Source: CAD feature listing. Evaluate the final solid. Frame: model axes, mm. A direction names the side the tool comes from. Give positions to 0.01 mm unless a question says otherwise; leave off trailing zeros. Order: outer loops, then holes, each group sorted by start corner. A loop starts at its lowest first (then second) coordinate and runs counter-clockwise, first axis right, second up. Notation, with made-up numbers: (-15, -1.5) - (14, -1.5) arc R14 cw to (14, 9.5) - close; hole circle Ø4 at (-27.75, 89). An arc over 180 degrees is marked (long way). Use CSV: the item, a comma, the result in double quotes.
```python
from build123d import *

# Parameters (mm, degrees)
CHAMFER_SIZE    = 0.5
CHAMFER001_SIZE = 1
CHAMFER002_SIZE = 0.5
SKETCH001_W     = 2
SKETCH001_H     = 21.821188
POCKET_DEPTH    = 18.001


with BuildPart() as part:
    # Sketch → Revolution (revolve)
    with BuildSketch(Plane.XZ):
        Polygon((12.9, 0), (17.9, 0), (17.9, 12), (14.9, 12), (14.9, 18), (12.9, 18), align=None)
    revolve(axis=Axis((0, 0, 0), (0, 0, 1)))

    # Chamfer
    chamfer_edges = [part.edges().sort_by_distance(p)[0] for p in [
        (-14.9, 0, 12),
    ]]
    chamfer(chamfer_edges, length=CHAMFER_SIZE)

    # Chamfer001
    chamfer001_edges = [part.edges().sort_by_distance(p)[0] for p in [
        (-14.9, 0, 18),
    ]]
    chamfer(chamfer001_edges, length=CHAMFER001_SIZE)

    # Chamfer002
    chamfer002_edges = [part.edges().sort_by_distance(p)[0] for p in [
        (-12.9, 0, 0),
    ]]
    chamfer(chamfer002_edges, length=CHAMFER002_SIZE)

    # Sketch001 (on Face4 of Chamfer002) → Pocket (cut, through all)
    with BuildSketch(Plane(origin=(0, 0, 0), x_dir=(1, 0, 0), z_dir=(0, 0, -1))):
        with Locations((-0.050035, -17.700875)):
            Rectangle(SKETCH001_W, SKETCH001_H)
    extrude(amount=-POCKET_DEPTH, mode=Mode.SUBTRACT)


solid = part.part
```
Item 1: Section A-A on x = 0. Return the cut outline in (y, z), then the cut area to 3 significant figures.
Filled in:
outline,"(-17.9, 0) - (-13.4, 0) - (-12.9, 0.5) - (-12.9, 18) - (-13.9, 18) - (-14.9, 17) - (-14.9, 12.5) - (-15.4, 12) - (-17.9, 12) - close"
area,"71.5 mm2"
Item 2: Section B-B on z = 4. Return the cut outline in (x, y).
Filled in:
outline,"(-1.05, 12.86) - (-1.05, 17.87) arc R17.9 ccw (long way) to (0.95, 17.87) - (0.95, 12.86) arc R12.9 cw (long way) to start"
Item 3: First-contact query: pin 1 (1 mm diameter, centred on y = 13.5, z = 10, fed in from -X); pin 2 (4 mm diameter, centred on x = -9.5, y = -6, fed in from -Z); pin 3 (6 mm diameter, centred on y = 9.5, z = 14, fed in from -X). Flat tips, straight axial feed; report the tip coordinate or a pass-through.
Filled in:
pin 1,"stops at x = -12.3"
pin 2,"stops at z = 0.16"
pin 3,"stops at x = -16.36"
Item 4: Set-up query: faces 1 (the cylindrical face through (-0.5, -12.89, 9.13)), 2 (the flat face through (0.95, 15, 7)), 3 (the flat face through (-15, -5, 12)). Return all of +Z, -Z, +X, -X, +Y, -Y with unobstructed straight access to the full face (end or side cutting, diameter ignored); none if empty.
Filled in:
face 1,"+Z, -Z"
face 2,"+Z, -Z, +Y"
face 3,"+Z"
Item 5: Material intervals for line 1 (X direction, y = 0, z = 7.5); line 2 (X direction, y = 0, z = 14); line 3 (Y direction, x = 0, z = 8.25), sorted ascending. Write a range as from..to.
Filled in:
line 1,"x = -17.9..-12.9, 12.9..17.9"
line 2,"x = -14.9..-12.9, 12.9..14.9"
line 3,"y = -17.9..-12.9"
Item 6: Section C-C on z = 13.75. Return the cut outline in (x, y).
Filled in:
outline,"(-1.05, 12.86) - (-1.05, 14.86) arc R14.9 ccw (long way) to (0.95, 14.87) - (0.95, 12.86) arc R12.9 cw (long way) to start"
Item 7: Mould query, pull axis X, two halves, no side actions, for faces 4 (the flat face through (-2.6, 13.3, 0)), 5 (the conical face through (-0.599, -15.023, 12.365)), 6 (the flat face through (-1.05, 15, 7)). Classes: released by +X, released by -X, zero draft, split by the parting line, or undercut.
Filled in:
face 4,"zero draft"
face 5,"split by the parting line"
face 6,"undercut"
